from build123d import *

# Parameters (mm, degrees)
ESBO_O2_R                = 1.5
RESSALTO_EXTRUS_O1_DEPTH = 1.52
ESBO_O3_W                = 9.002839431
ESBO_O3_H                = 14.464026403
RESSALTO_EXTRUS_O2_DEPTH = 11
ESBO_O4_W                = 2.6
ESBO_O4_H                = 21
ESBO_O4_H_2              = 26
ESBO_O4_H_3              = 15.7
RESSALTO_EXTRUS_O3_DEPTH = 8.4
CORTE_EXTRUS_O1_DEPTH    = 12
ESBO_O6_R                = 3.501419715
ESBO_O6_R_2              = 1
CORTE_EXTRUS_O2_DEPTH    = 12
FILETE1_R                = 1
FILETE2_R                = 0.5
ESBO_O7_W                = 12.143418905
ESBO_O7_H                = 16.377735741
RESSALTO_EXTRUS_O4_DEPTH = 10.8
CORTE_EXTRUS_O3_DEPTH    = 10
ESBO_O10_W               = 9.554785471
ESBO_O10_H               = 35.312042965
RESSALTO_EXTRUS_O5_DEPTH = 7
FILETE3_R                = 1
ESBO_O11_W               = 10.159902464
ESBO_O11_H               = 35.738148994
RESSALTO_EXTRUS_O6_DEPTH = 3


with BuildPart() as part:
    # Esboço2 → Ressalto-extrusão1 (new body)
    with BuildSketch(Plane.XY):
        with BuildLine():
            Line((26.8, -30.777402322), (25.217451408, -32.359950915))
            Line((25.217451408, -32.359950915), (13.7271729, -32.359950915))
            Line((13.7271729, -32.359950915), (11.181461411, -34.905662403))
            Line((11.181461411, -34.905662403), (-21.61825292, -34.905662403))
            Line((-21.61825292, -34.905662403), (-24.163964409, -32.359950915))
            Line((-24.163964409, -32.359950915), (-25.8, -32.359950915))
            ThreePointArc((-25.8, -32.359950915), (-26.507106781, -32.067057696), (-26.8, -31.359950915))
            Line((-26.8, -31.359950915), (-26.8, 33.15))
            ThreePointArc((-26.8, 33.15), (-26.507106781, 33.857106781), (-25.8, 34.15))
            Line((-25.8, 34.15), (25.8, 34.15))
            ThreePointArc((25.8, 34.15), (26.507106781, 33.857106781), (26.8, 33.15))
            Line((26.8, 33.15), (26.8, -30.777402322))
        make_face()
        with Locations((24.189792897, 18.770096718)):
            Circle(ESBO_O2_R, mode=Mode.SUBTRACT)
        with Locations((-24.163964409, 19.991194307)):
            Circle(ESBO_O2_R, mode=Mode.SUBTRACT)
        with Locations((-19.149057151, -32.359950915)):
            Circle(ESBO_O2_R, mode=Mode.SUBTRACT)
        with Locations((8.800152978, -32.359950915)):
            Circle(ESBO_O2_R, mode=Mode.SUBTRACT)
    extrude(amount=RESSALTO_EXTRUS_O1_DEPTH)

    # Esboço3 → Ressalto-extrusão2 (add)
    with BuildSketch(Plane.XY.offset(1.52)):
        with Locations((-19.353564393, 28.321014274)):
            Rectangle(ESBO_O3_W, ESBO_O3_H)
    extrude(amount=RESSALTO_EXTRUS_O2_DEPTH)

    # Esboço4 → Ressalto-extrusão3 (add)
    with BuildSketch(Plane.XY.offset(1.52)):
        with Locations((24.334460994, -20.701802403)):
            Rectangle(ESBO_O4_W, ESBO_O4_H)
        with Locations((24.334460994, 3.658197597)):
            Rectangle(ESBO_O4_W, ESBO_O4_H_2)
        with Locations((-24.092015344, -2.684387248)):
            Rectangle(ESBO_O4_W, ESBO_O4_H)
        with Locations((-24.092015344, -23.409860345)):
            Rectangle(ESBO_O4_W, ESBO_O4_H_3)
    extrude(amount=RESSALTO_EXTRUS_O3_DEPTH)

    # Esboço5 → Corte-extrusão1 (cut)
    with BuildSketch(Plane.XZ.offset(-21.089001072)):
        with BuildLine():
            Line((-14.852144677, 7.52), (-14.852144677, 12.52))
            Line((-14.852144677, 12.52), (-23.854984108, 12.52))
            Line((-23.854984108, 12.52), (-23.854984108, 7.52))
            ThreePointArc((-23.854984108, 7.52), (-19.353564393, 12.021419715), (-14.852144677, 7.52))
        make_face()
    extrude(amount=-CORTE_EXTRUS_O1_DEPTH, mode=Mode.SUBTRACT)

    # Esboço6 → Corte-extrusão2 (cut)
    with BuildSketch(Plane.XZ.offset(-35.553027475)):
        with Locations(Location((-19.353564393, 7.52, 0), (0, 0, 270))):
            Circle(ESBO_O6_R)
        with Locations(Location((-19.353564393, 7.52, 0), (0, 0, 270))):
            Circle(ESBO_O6_R_2, mode=Mode.SUBTRACT)
    extrude(amount=CORTE_EXTRUS_O2_DEPTH, mode=Mode.SUBTRACT)

    # Filete1
    filete1_edges = [part.edges().sort_by_distance(p)[0] for p in [
        (-19.353564393, 35.553027475, 8.52),
    ]]
    fillet(filete1_edges, radius=FILETE1_R)

    # Filete2
    filete2_edges = [part.edges().sort_by_distance(p)[0] for p in [
        (-14.852144677, 34.321014274, 12.52),
        (-23.854984108, 34.321014274, 12.52),
    ]]
    fillet(filete2_edges, radius=FILETE2_R)

    # Esboço7 → Ressalto-extrusão4 (add)
    with BuildSketch(Plane.XY.offset(1.52)):
        with Locations((11.324094847, 32.5040773)):
            Rectangle(ESBO_O7_W, ESBO_O7_H)
    extrude(amount=RESSALTO_EXTRUS_O4_DEPTH)

    # Esboço9 → Corte-extrusão3 (cut)
    with BuildSketch(Plane(origin=(0, 40.69294517, 0), x_dir=(1, 0, 0), z_dir=(0, 1, 0))):
        with BuildLine():
            Line((6.952385394, -2.72), (15.695804299, -2.72))
            ThreePointArc((15.695804299, -2.72), (16.04935769, -2.866446609), (16.195804299, -3.22))
            Line((16.195804299, -3.22), (16.195804299, -8.912893219))
            ThreePointArc((16.195804299, -8.912893219), (16.157744065, -9.104234935), (16.04935769, -9.266446609))
            Line((16.04935769, -9.266446609), (14.342250908, -10.973553391))
            ThreePointArc((14.342250908, -10.973553391), (14.180039234, -11.081939766), (13.988697518, -11.12))
            Line((13.988697518, -11.12), (8.659492175, -11.12))
            ThreePointArc((8.659492175, -11.12), (8.468150459, -11.081939766), (8.305938785, -10.973553391))
            Line((8.305938785, -10.973553391), (6.598832004, -9.266446609))
            ThreePointArc((6.598832004, -9.266446609), (6.490445628, -9.104234935), (6.452385394, -8.912893219))
            Line((6.452385394, -8.912893219), (6.452385394, -3.22))
            ThreePointArc((6.452385394, -3.22), (6.598832004, -2.866446609), (6.952385394, -2.72))
        make_face()
        with BuildLine():
            Line((14.024094847, -8.17), (8.624094847, -8.17))
            ThreePointArc((8.624094847, -8.17), (8.411962812, -8.082132034), (8.324094847, -7.87))
            Line((8.324094847, -7.87), (8.324094847, -5.97))
            ThreePointArc((8.324094847, -5.97), (8.411962812, -5.757867966), (8.624094847, -5.67))
            Line((8.624094847, -5.67), (14.024094847, -5.67))
            ThreePointArc((14.024094847, -5.67), (14.236226881, -5.757867966), (14.324094847, -5.97))
            Line((14.324094847, -5.97), (14.324094847, -7.87))
            ThreePointArc((14.324094847, -7.87), (14.236226881, -8.082132034), (14.024094847, -8.17))
        make_face(mode=Mode.SUBTRACT)
    extrude(amount=-CORTE_EXTRUS_O3_DEPTH, mode=Mode.SUBTRACT)

    # Esboço10 → Ressalto-extrusão5 (add)
    with BuildSketch(Plane.XY.offset(1.52)):
        with Locations((-10.358620196, -12.664154249)):
            Rectangle(ESBO_O10_W, ESBO_O10_H)
    extrude(amount=RESSALTO_EXTRUS_O5_DEPTH)

    # Filete3
    filete3_edges = [part.edges().sort_by_distance(p)[0] for p in [
        (-5.58122746, -12.664154249, 8.52),
        (-10.358620195, 4.991867234, 8.52),
        (-15.136012931, -12.664154249, 8.52),
        (-10.358620195, -30.320175731, 8.52),
    ]]
    fillet(filete3_edges, radius=FILETE3_R)

    # Esboço11 → Ressalto-extrusão6 (add)
    with BuildSketch(Plane.XY.offset(1.52)):
        with Locations((-10.332437347, -12.5521927)):
            Rectangle(ESBO_O11_W, ESBO_O11_H)
    extrude(amount=RESSALTO_EXTRUS_O6_DEPTH)


solid = part.part
Part model, mm, in its own coordinate system. A direction names the side the tool comes from. Coordinates: 2 decimals unless noted, no trailing zeros. Loops run counter-clockwise (first coordinate to the right, second up) from the corner with the lowest first, then second, coordinate; pieces in that order, holes last. Notation, with made-up numbers: M 84,32 L 122,32 A20 cw 122,71 Z; hole C 13,85 d5. An arc over 180 degrees is marked long. Use a Markdown table: item, result. Add a question column.
Q1. Mould opens along Y. For faces 1 (the cylindrical face through (24.88, 17.44, 0.75)), 2 (the flat face through (-10, -30.421, 3)), 3 (the cylindrical face through (-25.663, 20.057, 0.749)), 4 (the flat face through (-25.392, -24, 6)) say: +Y half, -Y half, draft (parallel to the pull), parting line (faces both ways), or undercut.
Q2. Cut at A-A (x = -12). Write the cut outline in (y, z), and give its area (3 significant figures).
Q3. Which spindle directions (+Z, -Z, +X, -X, +Y, -Y) get a long thin tool onto all of the face, cutting with end or side? Do faces 5 (the cylindrical face through (-15.882, 29.637, 7.976)), 6 (the flat face through (-24, -31.26, 6)), 7 (the flat face through (-25.392, -3, 6)), 8 (the flat face through (-15.136, -13, 6)), 9 (the flat face through (-14.852, 28, 4)). Say none if no direction does.
Q4. Cut at B-B (y = -6.5). Write the cut outline in (x, z), and give its area (3 significant figures).
Q5. Pin check, flat tips, straight feed: P1, Ø6, axis at x = -11, z = 10.5, coming from the +Y side; P2, Ø5, axis at x = 11, y = 38, coming from the -Z side; P3, Ø7, axis at x = 12, y = 34, coming from the +Z side. Stop position of each tip, or through.
Q6. Probe L1, parallel to X at y = -24.5, z = 3.75; L2, parallel to Y at x = -23, z = 2.75; L3, parallel to X at y = 37.5, z = 3.25. List the from-to ranges inside material, lowest first.
Worked out:
| question | item | result |
|---|---|---|
| 1 | face 1 | undercut |
| 1 | face 2 | -Y half |
| 1 | face 3 | undercut |
| 1 | face 4 | draft |
| 2 | outline | M -34.91,0 L 34.15,0 L 34.15,1.52 L 5.32,1.52 L 5.32,4.52 L 4.99,4.52 L 4.99,7.52 A1 ccw 3.99,8.52 L -29.32,8.52 A1 ccw -30.32,7.52 L -30.32,4.52 L -30.42,4.52 L -30.42,1.52 L -34.91,1.52 Z |
| 2 | area | 353 mm2 |
| 3 | face 5 | +Y |
| 3 | face 6 | +Z, +X, -X, -Y |
| 3 | face 7 | +Z, -X, +Y, -Y |
| 3 | face 8 | +Z, -Y |
| 3 | face 9 | +Z, +Y |
| 4 | outline | M -26.8,0 L 26.8,0 L 26.8,1.52 L 25.63,1.52 L 25.63,9.92 L 23.03,9.92 L 23.03,1.52 L -5.25,1.52 L -5.25,4.52 L -5.58,4.52 L -5.58,7.52 A1 ccw -6.58,8.52 L -14.14,8.52 A1 ccw -15.14,7.52 L -15.14,4.52 L -15.41,4.52 L -15.41,1.52 L -22.79,1.52 L -22.79,9.92 L -25.39,9.92 L -25.39,1.52 L -26.8,1.52 Z |
| 4 | area | 193 mm2 |
| 5 | P1 | stops at y = 4.99 |
| 5 | P2 | stops at z = 1.52 |
| 5 | P3 | stops at z = 12.32 |
| 6 | L1 | x = -25.39 to -22.79, -15.41 to -5.25, 23.03 to 25.63 |
| 6 | L2 | y = -31.26 to -15.56, -13.18 to 7.82, 21.09 to 35.55 |
| 6 | L3 | x = 5.25 to 6.45, 16.2 to 17.4 |
